Input: part model. Units: mm. Frame: model coordinates. A direction names the side the tool comes from. Round coordinates to 2 decimals unless told otherwise and drop trailing zeros.
(1) Access query for faces 1 (the face through (6.1, -6.46, 1.6)), 2 (the face through (16.9, -2.015, 1.6)), 3 (the face through (17.731, 0.2, 1.6)), 4 (the face through (12.175, -6.8, 1.6)), 5 (the face through (16.62, -4.4, 1.6)). Directions: +Z, -Z, +X, -X, +Y, -Y. A direction counts if a zero-diameter tool reaches every point of the face in a straight line with its end or side. Return the directions, or none.
(2) First-contact query: pin 1 Ø0.6 at (x, z) = (6.5, 1.5) entering from -Y; pin 2 Ø0.6 at (y, z) = (3.5, 2) entering from +X; pin 3 Ø0.6 at (x, z) = (17, 1.5) entering from -Y. Flat tips, straight axial feed; report the tip coordinate or a pass-through.
(3) Draft query along X for faces 6 (the face through (7.73, -6.8, 1.6)), 7 (the face through (16.62, 4, 1.6)), 8 (the face through (14.6, -6.46, 1.6)). Return one class per face: released by +X, released by -X, zero draft, split by the parting line, or undercut.
(4) Line query: line 1 (X direction, y = -7, z = 1.25); line 2 (Y direction, x = 16.75, z = 1.85); line 3 (Y direction, x = 16.5, z = 1.15). Output: solid intervals per line, ascending.
from build123d import *

# Parameters (mm, degrees)
BOSS_EXTRUDE1_DEPTH = 3.175
SKETCH2_W           = 12.7
SKETCH2_H           = 3.175
BOSS_EXTRUDE2_DEPTH = 3.175
SKETCH3_W           = 3.175
SKETCH3_H           = 12.7
BOSS_EXTRUDE3_DEPTH = 3.175
CUT_EXTRUDE1_REACH  = 5.175
FILLET1_R           = 0.508
SCALE1_SCALE        = 0.35


with BuildPart() as part:
    # Sketch1 → Boss-Extrude1 (new body)
    with BuildSketch(Plane.XY):
        with BuildLine():
            Line((22.86, -12.7), (-12.7, -12.7))
            add(Edge.make_bspline(
                [(22.86, 22.86), (14.060256121, 1.487897552), (8.672102448, -3.900256121), (-12.7, -12.7)],
                knots=[0, 0, 0, 0, 1, 1, 1, 1], degree=3))
            Line((22.86, 22.86), (22.86, -12.7))
        make_face()
    extrude(amount=BOSS_EXTRUDE1_DEPTH)

    # Sketch2 → Boss-Extrude2 (add)
    with BuildSketch(Plane.XZ.offset(12.7)):
        with Locations((3.81, 1.5875)):
            Rectangle(SKETCH2_W, SKETCH2_H)
    extrude(amount=BOSS_EXTRUDE2_DEPTH)

    # Sketch3 → Boss-Extrude3 (add)
    with BuildSketch(Plane(origin=(22.86, 0, 0), x_dir=(0, 0, -1), z_dir=(1, 0, 0))):
        with Locations((-1.5875, 6.35)):
            Rectangle(SKETCH3_W, SKETCH3_H)
    extrude(amount=BOSS_EXTRUDE3_DEPTH)

    # Sketch4 → Cut-Extrude1 (cut, up to next)
    with BuildSketch(Plane.XY.offset(3.175), mode=Mode.PRIVATE) as cut_extrude1_sk1:
        with BuildLine():
            Line((-3.556, -11.938), (-3.556, -12.7))
            Line((-3.556, -12.7), (-2.54, -12.7))
            Line((-2.54, -12.7), (-2.54, -11.938))
            ThreePointArc((-2.54, -11.938), (-3.048, -11.43), (-3.556, -11.938))
        make_face()
    cut_extrude1_tool1 = extrude(cut_extrude1_sk1.sketch, amount=-CUT_EXTRUDE1_REACH, mode=Mode.PRIVATE) & part.part
    add(cut_extrude1_tool1.solids().sort_by_distance((-3.048, -12.113972, 3.175))[0], mode=Mode.SUBTRACT)
    # Sketch4 → Cut-Extrude1 (cut, up to next)
    with BuildSketch(Plane.XY.offset(3.175), mode=Mode.PRIVATE) as cut_extrude1_sk2:
        with BuildLine():
            Line((10.16, -11.938), (10.16, -12.7))
            Line((10.16, -12.7), (11.176, -12.7))
            Line((11.176, -12.7), (11.176, -11.938))
            ThreePointArc((11.176, -11.938), (10.668, -11.43), (10.16, -11.938))
        make_face()
    cut_extrude1_tool2 = extrude(cut_extrude1_sk2.sketch, amount=-CUT_EXTRUDE1_REACH, mode=Mode.PRIVATE) & part.part
    add(cut_extrude1_tool2.solids().sort_by_distance((10.668, -12.113972, 3.175))[0], mode=Mode.SUBTRACT)
    # Sketch4 → Cut-Extrude1 (cut, up to next)
    with BuildSketch(Plane.XY.offset(3.175), mode=Mode.PRIVATE) as cut_extrude1_sk3:
        with BuildLine():
            Line((22.098, -1.016), (22.86, -1.016))
            Line((22.86, -1.016), (22.86, 0))
            Line((22.86, 0), (22.098, 0))
            ThreePointArc((22.098, 0), (21.59, -0.508), (22.098, -1.016))
        make_face()
    cut_extrude1_tool3 = extrude(cut_extrude1_sk3.sketch, amount=-CUT_EXTRUDE1_REACH, mode=Mode.PRIVATE) & part.part
    add(cut_extrude1_tool3.solids().sort_by_distance((22.273972, -0.508, 3.175))[0], mode=Mode.SUBTRACT)
    # Sketch4 → Cut-Extrude1 (cut, up to next)
    with BuildSketch(Plane.XY.offset(3.175), mode=Mode.PRIVATE) as cut_extrude1_sk4:
        with BuildLine():
            Line((22.098, 12.7), (22.86, 12.7))
            Line((22.86, 12.7), (22.86, 13.716))
            Line((22.86, 13.716), (22.098, 13.716))
            ThreePointArc((22.098, 13.716), (21.59, 13.208), (22.098, 12.7))
        make_face()
    cut_extrude1_tool4 = extrude(cut_extrude1_sk4.sketch, amount=-CUT_EXTRUDE1_REACH, mode=Mode.PRIVATE) & part.part
    add(cut_extrude1_tool4.solids().sort_by_distance((22.273972, 13.208, 3.175))[0], mode=Mode.SUBTRACT)

    # Fillet1
    fillet1_edges = [part.edges().sort_by_distance(p)[0] for p in [
        (22.86, 13.716, 1.5875),
        (26.035, 12.7, 1.5875),
        (26.035, 0, 1.5875),
        (22.86, -1.016, 1.5875),
        (22.86, -12.7, 1.5875),
        (11.176, -12.7, 1.5875),
        (10.16, -15.875, 1.5875),
        (-2.54, -15.875, 1.5875),
        (-3.556, -12.7, 1.5875),
        (-12.7, -12.7, 1.5875),
        (22.86, 22.86, 1.5875),
    ]]
    fillet(fillet1_edges, radius=FILLET1_R)


with BuildPart() as part_1:
    # Scale1: scaled about (13.259441719, -3.099441698, 1.5875)
    add(part.part.scale(SCALE1_SCALE).moved(Location((8.618637117, -2.014637104, 1.031875))))


solid = part_1.part
Reported:
1. face 1: +Z, -Z, -X, -Y
1. face 2: +Z, -Z, +X
1. face 3: +Z, -Z, +X, +Y, -Y
1. face 4: +Z, -Z, -Y
1. face 5: +Z, -Z, +X, -Y
2. pin 1: stops at y = -6.46
2. pin 2: stops at x = 16.62
2. pin 3: stops at y = -2.01
3. face 6: undercut
3. face 7: released by +X
3. face 8: zero draft
4. line 1: x = 7.73 to 12.17
4. line 2: y = -2.01 to 2.43
4. line 3: y = -6.45 to -2.38, -2.01 to 2.43, 2.8 to 5.27
